For this review, take the finished solid that the model builds, in its own axes (mm). A direction names the side the tool comes from. Round coordinates to 2 decimals unless told otherwise and drop trailing zeros. Write each loop counter-clockwise with the first axis right and the second up, starting at its lowest first coordinate (ties: lowest second). Pieces come first, ordered by that corner, then holes. Notation, with made-up numbers: (75.25, 87) -> (89.25, 87) arc R15 ccw to (89.25, 96) -> close; hole circle Ø8 at (25, 42.25). An arc over 180 degrees is marked (long way). Write each question's results on one line, items separated by ' | '. Start each with the question number.
Item 1: Add section C-C (x = 34). State the section outline as (y, z) points, plus the area to 3 significant figures.
Item 2: Add section D-D (x = 333.5). State the section outline as (y, z) points (3 decimals).
Item 3: Add section A-A (x = 150). State the section outline as (y, z) points, plus the area to 3 significant figures.
Item 4: Clearance check with flat-ended pins moving along their axes: pin 1 (4 mm diameter, centred on x = 82, z = 164, fed in from -Y); pin 2 (1.5 mm diameter, centred on x = 63, y = -77.5, fed in from -Z); pin 3 (8 mm diameter, centred on y = 161.5, z = -3, fed in from +X). State where each tip first meets the part, or that it passes through.
Item 5: Tool access review of faces 4 (the flat face through (216, 300, 0)), 5 (the cylindrical face through (152.858, 189.564, -64.937)), 6 (the flat face through (70, 186, 101)): name each direction out of +Z, -Z, +X, -X, +Y, -Y from which nothing blocks a thin tool from reaching the whole face with its end or side.
Item 6: The part is to be moulded in two halves that separate along X. For faces 1 (the flat face through (0, 44, 90)), 2 (the cylindrical face through (229.32, 214.6, -10.41)), 3 (the cylindrical face through (34.51, -63.08, 200.3)), say which applies: +X half, -X half, draft (parallel to the pull), parting line (faces both ways), or undercut.
Item 7: To check wall thickness, follow line 1 along Z through (x, y) = (150, 132); line 2 along X through (y, z) = (-197.5, -29); line 3 along Y through (x, z) = (342, 0). State the ranges of each line that lie inside material, in increasing order.
Item 8: Add section B-B (y = 181). State the section outline as (x, z) points, plus the area to 3 significant figures.
from build123d import *

# Parameters (mm, degrees)
BOSS_EXTRU_1_REACH      = 728.223
ESQUISSE3_R             = 80
ESQUISSE4_R             = 65
ENL_V_MAT_EXTRU_1_DEPTH = 280


with BuildPart() as part:
    # Esquisse1 → Révolution1 (revolve)
    with BuildSketch(Plane.XY, mode=Mode.PRIVATE) as r_volution1_sk:
        Polygon((0, 100), (440, 100), (440, 110), (280, 150), (100, 150), (100, 230), (70, 230), (70, 210), (0, 210), align=None)
    revolve(r_volution1_sk.sketch.rotate(Axis((0, 0, 0), (1, 0, 0)), 90), axis=Axis((0, 0, 0), (1, 0, 0)))

    # Esquisse3 → Boss.-Extru.1 (add, up to next)
    with BuildSketch(Plane(origin=(0, 300, 0), x_dir=(1, 0, 0), z_dir=(0, 1, 0)), mode=Mode.PRIVATE) as boss_extru_1_sk1:
        with Locations(Location((150, 0, 0), (0, 0, 270))):
            Circle(ESQUISSE3_R)
    boss_extru_1_tool1 = extrude(boss_extru_1_sk1.sketch, amount=-BOSS_EXTRU_1_REACH, mode=Mode.PRIVATE) - part.part
    add(boss_extru_1_tool1.solids().sort_by_distance((150, 300, 0))[0])

    # Esquisse4 → Enlèv. mat.-Extru.1 (cut)
    with BuildSketch(Plane(origin=(0, 300, 0), x_dir=(1, 0, 0), z_dir=(0, 1, 0))):
        with Locations(Location((150, 0, 0), (0, 0, 270))):
            Circle(ESQUISSE4_R)
    extrude(amount=-ENL_V_MAT_EXTRU_1_DEPTH, mode=Mode.SUBTRACT)


solid = part.part
Responses:
1) outline: circle Ø420 at (0, 0); hole circle Ø200 at (0, 0) | area: 107,000 mm^2
2) outline: circle Ø273.25 at (0, 0); hole circle Ø200 at (0, 0)
3) outline: (75.99, -65) arc R100 cw (long way) to (75.99, 65) -> (300, 65) -> (300, 80) -> (126.89, 80) arc R150 ccw (long way) to (126.89, -80) -> (300, -80) -> (300, -65) -> close | area: 37,500 mm^2
4) pin 1: stops at y = -163.27 | pin 2: stops at z = -195.47 | pin 3: stops at x = 230
5) face 4: +Z, -Z, +X, -X, +Y | face 5: +Y | face 6: -X
6) face 1: -X half | face 2: undercut | face 3: draft
7) line 1: z = -80 to -65, 65 to 80 | line 2: x = 0 to 100 | line 3: y = -134.5 to -100, 100 to 134.5
8) outline: (0, -106.48) -> (70, -106.48) -> (70, -141.91) -> (100, -141.91) -> (100, -62.45) arc R80 ccw (long way) to (100, 62.45) -> (100, 141.91) -> (70, 141.91) -> (70, 106.48) -> (0, 106.48) -> close; hole circle Ø130 at (150, 0) | area: 27,600 mm^2
